The listing builds one solid part. Answer for the finished solid, in the listing's coordinates (mm). A direction names the side the tool comes from. Coordinates: 2 decimals unless noted, no trailing zeros. Order: outer loops, then holes, each group sorted by start corner. A loop starts at its lowest first (then second) coordinate and runs counter-clockwise, first axis right, second up. Notation, with made-up numbers: (-9, -39.5) -> (28, -39.5) arc R23 ccw to (28, -27.5) -> close; hole circle Ø7 at (30, -25.5). An arc over 180 degrees is marked (long way). Answer in a Markdown table with one row per item.
```python
from build123d import *

# Parameters (mm, degrees)
F1_DEPTH = 63.5
F2_DEPTH = 50.8
F3_DEPTH = 15.875
F5_R     = 6.35


with BuildPart() as f1:
    # F0 (on Front) → F1 (new body, symmetric)
    with BuildSketch(Plane.XZ):
        Polygon((41.275, -9.525), (41.275, 9.525), (22.225, 9.525), (-41.275, 9.525), (-41.275, -9.525), align=None)
    extrude(amount=F1_DEPTH, both=True)

    # F0 (on Front) → F2 (join)
    with BuildSketch(Plane.XZ):
        with BuildLine():
            Line((22.225, 9.525), (41.275, 9.525))
            Line((41.275, 9.525), (41.275, 27.0002))
            ThreePointArc((41.275, 27.0002), (45.92468, 38.22552), (57.15, 42.8752))
            Line((57.15, 42.8752), (60.325, 42.8752))
            Line((60.325, 42.8752), (60.325, 61.9252))
            Line((60.325, 61.9252), (57.15, 61.9252))
            ThreePointArc((57.15, 61.9252), (32.454296, 51.695904), (22.225, 27.0002))
            Line((22.225, 27.0002), (22.225, 9.525))
        make_face()
        Polygon((60.325, 61.9252), (60.325, 42.8752), (74.941066, 42.8752), (85.725, 42.8752), (85.725, 61.9252), (74.941066, 61.9252), align=None)
    extrude(amount=F2_DEPTH)

    # F0 (on Front) → F3 (join)
    with BuildSketch(Plane.XZ):
        with BuildLine():
            Line((-41.275, 9.525), (22.225, 9.525))
            Line((22.225, 9.525), (22.225, 27.0002))
            ThreePointArc((22.225, 27.0002), (32.454296, 51.695904), (57.15, 61.9252))
            add(Edge.make_bspline(
                [(-41.275, 9.525), (-41.235335, 51.891662), (10.656322, 64.555697), (57.15, 61.9252)],
                knots=[0, 0, 0, 0, 111.504536, 111.504536, 111.504536, 111.504536], degree=3))
        make_face()
    extrude(amount=F3_DEPTH)

    # F0 (on Front) → F4 (revolve)
    with BuildSketch(Plane.XZ):
        Polygon((85.725, 42.8752), (85.725, 38.1), (111.125, 38.1), (111.125, 66.675), (85.725, 66.675), (85.725, 61.9252), align=None)
    revolve(axis=Axis((85.725, 0, 52.3875), (0, 0, 1)))

    # F5
    f5_edges = [f1.edges().sort_by_distance(p)[0] for p in [
        (-41.275, -63.5, 0),
        (41.275, -63.5, 0),
        (41.275, 63.5, 0),
        (-41.275, 63.5, 0),
    ]]
    fillet(f5_edges, radius=F5_R)


solid = f1.part
```
(1) Find the intervals of material crossed by line 1 along X through (y, z) = (-47, 11) (3 decimals); line 2 along Y through (x, z) = (-19.5, 10) (3 decimals); line 3 along Z through (x, y) = (41, 21.5) (3 decimals), in increasing order. Write a range as from..to.
Check values:
| item | result |
|---|---|
| line 1 | 22.225..41.275 |
| line 2 | -15.875..0 |
| line 3 | -9.525..9.525 |
(2) A cutting plane is placed at C-C, the plane x = 94.5. Determine the outline of the cut face in (y, z) (3 decimals), then the cut area to 3 significant figures.
Check values:
| item | result |
|---|---|
| outline | (-23.836, 38.1) -> (23.836, 38.1) -> (23.836, 66.675) -> (-23.836, 66.675) -> close |
| area | 1,360 mm² |
(3) Which of the six approach directions +Z, -Z, +X, -X, +Y, -Y give full straight-line access (tool end or side, diameter ignored) to faces 1 (the flat face through (1, 31, 9.525)), 2 (the flat face through (-4, -15.875, 31)), 3 (the flat face through (46, -50.8, 42)), 4 (the flat face through (68, -31, 42.875))?
Check values:
| item | result |
|---|---|
| face 1 | +Z, +X, -X, +Y |
| face 2 | +Z, -X, -Y |
| face 3 | +Z, +X, -X, -Y |
| face 4 | -Z, -Y |
(4) Flat-ended cylindrical pins translate along their axes: pin 1 (12 mm diameter, centred on y = -8, z = 33, fed in from +X); pin 2 (11 mm diameter, centred on y = 0, z = 13.5, fed in from +X) (3 decimals); pin 3 (5 mm diameter, centred on y = -40, z = 20.5, fed in from -X) (3 decimals); pin 4 (3 mm diameter, centred on x = 44.5, y = 34, fed in from -Z). Find the tip coordinate at first contact, or state that the pin passes through.
Check values:
| item | result |
|---|---|
| pin 1 | x = 110.66 |
| pin 2 | x = 41.275 |
| pin 3 | x = 22.225 |
| pin 4 | through |
(5) A cutting plane is placed at A-A, the plane y = 12. Determine the outline of the cut face in (x, z) (3 decimals), then the cut area to 3 significant figures.
Check values:
| item | result |
|---|---|
| outline | (-41.275, -9.525) -> (41.275, -9.525) -> (41.275, 9.525) -> (-41.275, 9.525) -> close; (63.338, 38.1) -> (108.112, 38.1) -> (108.112, 66.675) -> (63.338, 66.675) -> close |
| area | 2,850 mm² |
(6) A cutting plane is placed at B-B, the plane y = 32.5. Determine the outline of the cut face in (x, z) (3 decimals).
Check values:
| item | result |
|---|---|
| outline | (-41.275, -9.525) -> (41.275, -9.525) -> (41.275, 9.525) -> (-41.275, 9.525) -> close |
